Geometry check sheet. Reference: the model listing, model coordinates, mm. Face numbers are marked on the shaded views. A direction names the side the tool comes from. Coordinates: 2 decimals unless noted, no trailing zeros. Write each loop counter-clockwise with the first axis right and the second up, starting at its lowest first coordinate (ties: lowest second). Pieces come first, ordered by that corner, then holes. Notation, with made-up numbers: (21, 7.5) -> (32, 7.5) arc R20 ccw to (32, 40.5) -> close; hole circle Ø7 at (-27.75, 83.5). An arc over 180 degrees is marked (long way). Put each result on its own line as item: value. Start each with the question number.
from build123d import *

# Parameters (mm, degrees)
F0_R     = 3
F1_DEPTH = 10
F2_R     = 5
F3_D     = 6


with BuildPart() as f1:
    # F0 (on Top) → F1 (new body)
    with BuildSketch(Plane.XY):
        with BuildLine():
            Line((-40, -24), (-12.3693168769, -24))
            ThreePointArc((-12.3693168769, -24), (-27, 0), (-12.3693168769, 24))
            Line((-12.3693168769, 24), (-40, 24))
            Line((-40, 24), (-40, -24))
        make_face()
        with BuildLine():
            Line((15, 0), (15, -15))
            Line((15, -15), (3.96875, -15))
            Line((3.96875, -15), (-3.96875, -15))
            Line((-3.96875, -15), (-15, -15))
            Line((-15, -15), (-15, 15))
            Line((-15, 15), (-3.96875, 15))
            Line((-3.96875, 15), (3.96875, 15))
            Line((3.96875, 15), (15, 15))
            Line((15, 15), (15, 4.21875))
            Line((15, 4.21875), (25.9915753842, 7.3101305768))
            ThreePointArc((25.9915753842, 7.3101305768), (20.9171568122, 17.0725672028), (12.3693168769, 24))
            Line((12.3693168769, 24), (-12.3693168769, 24))
            ThreePointArc((-12.3693168769, 24), (-27, 0), (-12.3693168769, -24))
            Line((-12.3693168769, -24), (12.3693168769, -24))
            ThreePointArc((12.3693168769, -24), (23.0539753153, -14.0539753153), (27, 0))
            Line((27, 0), (15, 0))
        make_face()
        with BuildLine():
            Line((15, 4.21875), (15, 0))
            Line((15, 0), (27, 0))
            ThreePointArc((27, 0), (26.7467057352, 3.6896791614), (25.9915753842, 7.3101305768))
            Line((25.9915753842, 7.3101305768), (15, 4.21875))
        make_face()
        with BuildLine():
            ThreePointArc((25.9915753842, 7.3101305768), (26.7467057352, 3.6896791614), (27, 0))
            ThreePointArc((27, 0), (23.0539753153, -14.0539753153), (12.3693168769, -24))
            Line((12.3693168769, -24), (40, -24))
            Line((40, -24), (40, 24))
            Line((40, 24), (12.3693168769, 24))
            ThreePointArc((12.3693168769, 24), (20.9171568122, 17.0725672028), (25.9915753842, 7.3101305768))
        make_face()
        with Locations((32, 16)):
            Circle(F0_R, mode=Mode.SUBTRACT)
        with Locations((32, 16)):
            Circle(F0_R)
    extrude(amount=F1_DEPTH)

    # F2
    f2_edges = [f1.edges().sort_by_distance(p)[0] for p in [
        (40, 24, 5),
        (40, -24, 5),
        (-40, 24, 5),
        (-40, -24, 5),
    ]]
    fillet(f2_edges, radius=F2_R)

    # F3 (through all)
    with Locations(Plane(origin=(0, 0, 0), x_dir=(1, 0, 0), z_dir=(0, 0, -1))):
        with Locations((32, -16), (32, 16), (-32, -16), (-32, 16)):
            Hole(F3_D / 2)


solid = f1.part
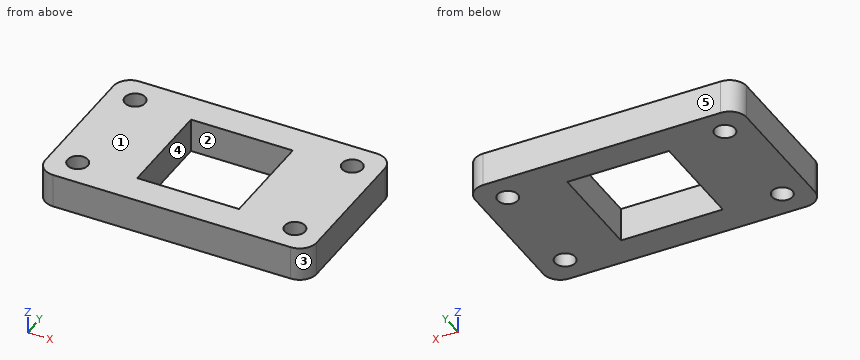
Item 1: Section check B-B, the plane z = 1.25. Enter the section's corners in (x, y), and give its area (3 significant figures).
Item 2: Section check A-A, the plane x = 32. Enter the section's corners in (y, z).
Item 3: Go/stop test with flat-tipped pins: P1, Ø3.5, axis at x = 32, y = 16, coming from the -Z side; P2, Ø12, axis at x = 29, y = -19, coming from the -Z side. Record where each tip stops, or that it passes through.
Item 4: Access from +Z, -Z, +X, -X, +Y, -Y to the whole of each face (thin tool, end or side, straight path). Record for the marked faces 4 and 5.
Item 5: Section check D-D, the plane x = 9.5. Enter the section's corners in (y, z).
Item 6: Section check C-C, the plane y = -11. Enter the section's corners in (x, z).
Item 7: Mould release check, pull along X, two halves, no side actions. Record for the marked faces 1, 2 and 3: released by +X, released by -X, zero draft, split by the parting line, or undercut.
Item 8: Scan lines: line 1 along Y through (x, z) = (32, 6.5); line 2 along X through (y, z) = (16, 5.75); line 3 along X through (y, z) = (-1.5, 3.75). Record each from-to range of solid material in increasing order. Write a range as [from, to].
From the geometry:
1. outline: (-40, -19) arc R5 ccw to (-35, -24) -> (35, -24) arc R5 ccw to (40, -19) -> (40, 19) arc R5 ccw to (35, 24) -> (-35, 24) arc R5 ccw to (-40, 19) -> close; hole circle Ø6 at (-32, -16); hole circle Ø6 at (-32, 16); hole (-15, -15) -> (15, -15) -> (15, 15) -> (-15, 15) -> close; hole circle Ø6 at (32, -16); hole circle Ø6 at (32, 16)
1. area: 2,810 mm²
2. outline: (-24, 0) -> (-19, 0) -> (-19, 10) -> (-24, 10) -> close; (-13, 0) -> (13, 0) -> (13, 10) -> (-13, 10) -> close; (19, 0) -> (24, 0) -> (24, 10) -> (19, 10) -> close
3. P1: through
3. P2: z = 0
4. face 4: +Z, -Z
4. face 5: +Z, -Z, +X, -X, +Y
5. outline: (-24, 0) -> (-15, 0) -> (-15, 10) -> (-24, 10) -> close; (15, 0) -> (24, 0) -> (24, 10) -> (15, 10) -> close
6. outline: (-40, 0) -> (-15, 0) -> (-15, 10) -> (-40, 10) -> close; (15, 0) -> (40, 0) -> (40, 10) -> (15, 10) -> close
7. face 1: zero draft
7. face 2: undercut
7. face 3: released by +X
8. line 1: [-24, -19], [-13, 13], [19, 24]
8. line 2: [-40, -35], [-29, 29], [35, 40]
8. line 3: [-40, -15], [15, 40]
